```python
from build123d import *

# Parameters (mm, degrees)
ESQUISSE1_R        = 30.160422997
BOSS_EXTRU_1_DEPTH = 70


with BuildPart() as part:
    # Esquisse1 → Boss.-Extru.1 (new body)
    with BuildSketch(Plane.XY):
        Circle(ESQUISSE1_R)
    extrude(amount=BOSS_EXTRU_1_DEPTH)

    # Esquisse10 → Trou taraudé 1 Rc1 (revolve, cut)
    with BuildSketch(Plane(origin=(0.041525869, 0.498310425, 0), x_dir=(0, 1, 0), z_dir=(1, 0, 0))):
        Polygon((0, 0), (0, 18.515361263), (17.5005, 8), (17.5005, 0.1), (16.028262338, 0.1), (16.031384, 0), align=None)
    revolve(axis=Axis((0.041525869, 0.498310425, -6.35), (0, 0, 1)), mode=Mode.SUBTRACT)


solid = part.part
```
The model under review builds one solid part; all positions refer to its coordinate system, in mm. Coordinates: 2 decimals unless noted, no trailing zeros. Order: outer loops, then holes, each group sorted by start corner. A loop starts at its lowest first (then second) coordinate and runs counter-clockwise, first axis right, second up. Notation, with made-up numbers: M -12.5,5 L -3.5,5 A19 cw -3.5,40 Z; hole C 74.25,24.5 d11. An arc over 180 degrees is marked long. One line per question, with ' | ' between items.
(1) The part is to be moulded in two halves that separate along Z. For faces 1 (the face through (0, 0, 70)), 2 (the face through (13, -13, 0)), 3 (the face through (28.768, 9.059, 34.51)), 4 (the face through (17.126, -3.295, 3.995)), say which applies: +Z half, -Z half, draft (parallel to the pull), parting line (faces both ways), or undercut.
Geometry results:
face 1: +Z half | face 2: -Z half | face 3: draft | face 4: undercut
(2) Add section A-A, the plane z = 29.5. Write out the cut boundary in (x, y), then the cut area to 3 significant figures.
Geometry results:
outline: C 0,0 d60.32 | area: 2,860 mm²
(3) Insertion check: pin 1 (5 mm diameter, centred on y = -7.5, z = 33, fed in from +X); pin 2 (6 mm diameter, centred on x = 11, z = 17.5, fed in from +Y); pin 3 (8 mm diameter, centred on y = -10, z = 23, fed in from -X). Each pin has a flat end and moves straight along its axis. Give the tip position at first contact, or say it passes through.
Geometry results:
pin 1: stops at x = 29.74 | pin 2: stops at y = 29.08 | pin 3: stops at x = -29.56
(4) Add section B-B, the plane x = -26. Write out the cut boundary in (y, z), then the cut area to 3 significant figures.
Geometry results:
outline: M -15.29,0 L 15.29,0 L 15.29,70 L -15.29,70 Z | area: 2,140 mm²
(5) For probe 1 along X at (y, z) = (-13, 4); probe 2 along X at (y, z) = (13.5, 3.5); probe 3 along Y at (x, z) = (-6, 9), list the stretches that pass through material, from the lowest coordinate up. Write a range as from..to.
Geometry results:
probe 1: x = -27.21..-11.1, 11.18..27.21 | probe 2: x = -26.97..-11.67, 11.76..26.97 | probe 3: y = -29.56..-14.14, 15.14..29.56
